from build123d import *

# Parameters (mm, degrees)
SKETCH1_W           = 28
SKETCH1_H           = 3
SKETCH1_W_2         = 3
SKETCH1_H_2         = 25
BOSS_EXTRUDE1_DEPTH = 10
CUT_EXTRUDE1_DEPTH  = 31.347981811
BOSS_EXTRUDE2_DEPTH = 3


with BuildPart() as part:
    # Sketch1 → Boss-Extrude1 (new, symmetric)
    with BuildSketch(Plane.XY):
        Rectangle(SKETCH1_W, SKETCH1_H)
        with Locations((-12.5, 14)):
            Rectangle(SKETCH1_W_2, SKETCH1_H_2)
    extrude(amount=BOSS_EXTRUDE1_DEPTH, both=True)

    # Sketch3 → Cut-Extrude1 (cut, through all)
    with BuildSketch(Plane(origin=(0, 1.5, 0), x_dir=(1, 0, 0), z_dir=(0, 1, 0))):
        with BuildLine():
            Line((8, -3.25), (-2, -3.25))
            ThreePointArc((-2, -3.25), (-5.25, 0), (-2, 3.25))
            Line((-2, 3.25), (8, 3.25))
            ThreePointArc((8, 3.25), (11.25, 0), (8, -3.25))
        make_face()
    cut_extrude1 = extrude(amount=-CUT_EXTRUDE1_DEPTH, mode=Mode.SUBTRACT)

    # Mirror1: Cut-Extrude1 across plane
    add(cut_extrude1.mirror(Plane(origin=(-6.25, 6.25, 0), x_dir=(0, 0, 1), z_dir=(-0.7071067811865479, 0.7071067811865471, 0))), mode=Mode.SUBTRACT)

    # Sketch4 → Boss-Extrude2 (add)
    with BuildSketch(Plane.XY.offset(10)):
        Polygon((-11, 26.5), (-8, 26.5), (-8, 23.5), (11, 4.5), (14, 4.5), (14, 1.5), (-11, 1.5), align=None)
    boss_extrude2 = extrude(amount=-BOSS_EXTRUDE2_DEPTH)

    # Mirror2: Boss-Extrude2 across plane
    add(boss_extrude2.mirror(Plane.XY))


solid = part.part
Geometry: final body of the model. Coordinates: model frame, mm. A direction names the side the tool comes from. Give positions to 0.01 mm unless a question says otherwise; leave off trailing zeros. Write each loop counter-clockwise with the first axis right and the second up, starting at its lowest first coordinate (ties: lowest second). Pieces come first, ordered by that corner, then holes.
(1) Cut plane B-B, the plane z = 0. Return loops of the section in (x, y).
(2) Cut plane A-A, the plane y = 16.75. Return loops of the section in (x, z).
(3) Access query for faces 1 (the flat face through (-4, 9, 7)), 2 (the cylindrical face through (-12.48, 7.25, 0.07)), 3 (the flat face through (-8, 25, 9)), 4 (the flat face through (3, 0, -3.25)). Directions: +Z, -Z, +X, -X, +Y, -Y. A direction counts if a zero-diameter tool reaches every point of the face in a straight line with its end or side. Return the directions, or none.
(4) Cut plane D-D, the plane x = -9.5. Return loops of the section in (y, z).
(5) Cut plane C-C, the plane x = -4.75. Return loops of the section in (y, z), then the cut area to 3 significant figures.
(6) Mould query, pull axis X, two halves, no side actions, for faces 5 (the flat face through (1.4, 14.1, -8.5)), 6 (the cylindrical face through (-12.48, 23.75, -0.07)), 7 (the cylindrical face through (-5.25, 0.02, 0.07)). Classes: released by +X, released by -X, zero draft, split by the parting line, or undercut.
(7) First-contact query: P1, Ø0.9, axis at x = 12.5, z = -8.5, coming from the +Y side; P2, Ø0.9, axis at y = 24.5, z = -8.5, coming from the +X side; P3, Ø4, axis at y = 15.5, z = -3, coming from the +X side; P4, Ø10, axis at x = 11, y = 18.5, coming from the +Z side. Flat tips, straight axial feed; report the tip coordinate or a pass-through.
(8) Ray query, line 1 (Z direction, x = -10.25, y = 22.75); line 2 (X direction, y = 5.25, z = -2.5); line 3 (Y direction, x = 2.25, z = -5.25). Return the intervals inside material, ascending.
Values follow:
1. outline: (-14, -1.5) - (-5.25, -1.5) - (-5.25, 1.5) - (-11, 1.5) - (-11, 7.25) - (-14, 7.25) - close; (-14, 23.75) - (-11, 23.75) - (-11, 26.5) - (-14, 26.5) - close; (11.25, -1.5) - (14, -1.5) - (14, 1.5) - (11.25, 1.5) - close
2. outline: (-14, -10) - (-1.25, -10) - (-1.25, -7) - (-11, -7) - (-11, -3.25) - (-14, -3.25) - close; (-14, 3.25) - (-11, 3.25) - (-11, 7) - (-1.25, 7) - (-1.25, 10) - (-14, 10) - close
3. face 1: +X, +Y
3. face 2: +X, -X
3. face 3: +Z, -Z, +X, +Y
3. face 4: +Y, -Y
4. outline: (-1.5, -10) - (26.5, -10) - (26.5, -7) - (1.5, -7) - (1.5, 7) - (26.5, 7) - (26.5, 10) - (-1.5, 10) - close
5. outline: (-1.5, -10) - (20.25, -10) - (20.25, -7) - (1.5, -7) - (1.5, -1.73) - (-1.5, -1.73) - close; (-1.5, 1.73) - (1.5, 1.73) - (1.5, 7) - (20.25, 7) - (20.25, 10) - (-1.5, 10) - close
5. area: 162 mm2
6. face 5: released by +X
6. face 6: zero draft
6. face 7: undercut
7. P1: stops at y = 4.5
7. P2: stops at x = -8
7. P3: stops at x = -11
7. P4: passes through
8. line 1: z = -10 to -7, 7 to 10
8. line 2: x = -14 to -11
8. line 3: y = -1.5 to 1.5
